Design review of the part built by this model. Coordinates are the model's own, in mm. A direction names the side the tool comes from. Coordinates: 2 decimals unless noted, no trailing zeros. Loops run counter-clockwise (first coordinate to the right, second up) from the corner with the lowest first, then second, coordinate; pieces in that order, holes last. Notation, with made-up numbers: (17.5, 18.5) -> (48.5, 18.5) arc R15 cw to (48.5, 26.5) -> close; hole circle Ø8 at (49, -1). An arc over 180 degrees is marked (long way). Use a Markdown table: item, result. Add a question column.
Q1. Take a section at D-D on x = -8. Write out the cut boundary in (y, z).
Q2. Take a section at B-B on x = -14. Write out the cut boundary in (y, z).
Q3. Take a section at A-A on z = 6.75. Write out the cut boundary in (x, y).
Q4. For probe 1 along X at (y, z) = (15.5, 15.5); probe 2 along Y at (x, z) = (-25, 11.5); probe 3 along Z at (x, y) = (-20.5, 3), list the stretches that pass through material, from the lowest coordinate up.
Q5. Take a section at C-C on y = 17. Write out the cut boundary in (x, z).
Q6. Clearance check with flat-ended pins moving along their axes: pin 1 Ø7 at (x, y) = (-24.98, 24.2) entering from +Z; pin 2 Ø3 at (x, y) = (-2.5, 11) entering from +Z. State where each tip first meets the part, or that it passes through.
Q7. Draft analysis for pull direction X (two halves, no side actions). For faces 3 (the face through (-34, 15, 11)), 4 (the face through (-21.757, 29.261, 2.507)), 5 (the face through (-16, 33, 11)), 6 (the face through (0, 15, 13)), state which applies: pulls with the +X half, pulls with the -X half, needs draft (parallel to the pull), parting line crosses it, or undercut.
Q8. For faces 1 (the face through (-16, 31, 13)), 2 (the face through (-16, 16, 0)), list the 3-axis set-ups (+Z, -Z, +X, -X, +Y, -Y) from which the entire face can be reached by the end or side of a thin tool; tool diameter is ignored.
from build123d import *

# Parameters (mm, degrees)
ESQUISSE1_W             = 32
ESQUISSE1_H             = 31
BOSS_EXTRU_1_DEPTH      = 3
BOSS_EXTRU_2_DEPTH      = 20
BOSS_EXTRU_2_DEPTH_BACK = 3
ESQUISSE2_W             = 36
ESQUISSE2_H             = 35
ESQUISSE2_W_2           = 32
ESQUISSE2_H_2           = 31
ESQUISSE3_R             = 1.5
ENL_V_MAT_EXTRU_1_DEPTH = 52.429563482
ESQUISSE4_R             = 6
ENL_V_MAT_EXTRU_2_DEPTH = 1


with BuildPart() as part:
    # Esquisse1 → Boss.-Extru.1 (new body)
    with BuildSketch(Plane.XY):
        with Locations((-16, 15.5)):
            Rectangle(ESQUISSE1_W, ESQUISSE1_H)
    extrude(amount=BOSS_EXTRU_1_DEPTH)

    # Esquisse2 → Boss.-Extru.2 (add, two sides: drawn at the far end of the back side and taken through both)
    with BuildSketch(Plane.XY.offset(3).offset(-BOSS_EXTRU_2_DEPTH_BACK)):
        with Locations((-16, 15.5)):
            Rectangle(ESQUISSE2_W, ESQUISSE2_H)
        with Locations((-16, 15.5)):
            Rectangle(ESQUISSE2_W_2, ESQUISSE2_H_2, mode=Mode.SUBTRACT)
    extrude(amount=BOSS_EXTRU_2_DEPTH + BOSS_EXTRU_2_DEPTH_BACK)

    # Esquisse3 → Enlèv. mat.-Extru.1 (cut, through all)
    with BuildSketch(Plane.XY.offset(3)):
        with Locations((-24.982527988, 24.201823988)):
            Circle(ESQUISSE3_R)
        with Locations((-7.026522418, 6.806943593)):
            Circle(ESQUISSE3_R)
    extrude(amount=-ENL_V_MAT_EXTRU_1_DEPTH, mode=Mode.SUBTRACT)

    # Esquisse4 → Enlèv. mat.-Extru.2 (cut)
    with BuildSketch(Plane.XY.offset(3)):
        with Locations((-24.982527988, 24.201823988)):
            Circle(ESQUISSE4_R)
        with Locations((-7.026522418, 6.806943593)):
            Circle(ESQUISSE4_R)
    extrude(amount=-ENL_V_MAT_EXTRU_2_DEPTH, mode=Mode.SUBTRACT)


solid = part.part
Answer list:
| question | item | result |
|---|---|---|
| 1 | outline | (-2, 0) -> (5.67, 0) -> (5.67, 2) -> (0.89, 2) -> (0.89, 3) -> (0, 3) -> (0, 23) -> (-2, 23) -> close; (7.95, 0) -> (33, 0) -> (33, 23) -> (31, 23) -> (31, 3) -> (12.73, 3) -> (12.73, 2) -> (7.95, 2) -> close |
| 2 | outline | (-2, 0) -> (33, 0) -> (33, 23) -> (31, 23) -> (31, 3) -> (0, 3) -> (0, 23) -> (-2, 23) -> close |
| 3 | outline | (-34, -2) -> (2, -2) -> (2, 33) -> (-34, 33) -> close; hole (-32, 0) -> (0, 0) -> (0, 31) -> (-32, 31) -> close |
| 4 | probe 1 | -34 to -32, 0 to 2 |
| 4 | probe 2 | -2 to 0, 31 to 33 |
| 4 | probe 3 | 0 to 3 |
| 5 | outline | (-34, 0) -> (2, 0) -> (2, 23) -> (0, 23) -> (0, 3) -> (-32, 3) -> (-32, 23) -> (-34, 23) -> close |
| 6 | pin 1 | z = 2 |
| 6 | pin 2 | z = 3 |
| 7 | face 3 | pulls with the -X half |
| 7 | face 4 | undercut |
| 7 | face 5 | needs draft |
| 7 | face 6 | undercut |
| 8 | face 1 | +Z |
| 8 | face 2 | -Z, +X, -X, +Y, -Y |
